Design review of the part built by this model. Coordinates are the model's own, in mm. Face numbers are marked on the shaded views. Give positions to 0.01 mm unless a question says otherwise; leave off trailing zeros. Order: outer loops, then holes, each group sorted by start corner. A loop starts at its lowest first (then second) coordinate and runs counter-clockwise, first axis right, second up. Notation, with made-up numbers: M 33.25,3 L 53.25,3 A8 ccw 53.25,10 Z; hole C 65.25,-2.75 d10. An arc over 180 degrees is marked long. Answer as a JSON object with one key per item and string values.
from build123d import *

# Parameters (mm, degrees)
SKETCH1_R           = 20
SKETCH1_R_2         = 1.5
SKETCH1_R_3         = 2
BOSS_EXTRUDE1_DEPTH = 7
SKETCH2_R           = 3.25
CUT_EXTRUDE1_DEPTH  = 1.5


with BuildPart() as part:
    # Sketch1 → Boss-Extrude1 (new body)
    with BuildSketch(Plane(origin=(0, 0, 0), x_dir=(1, 0, 0), z_dir=(0, 1, 0))):
        with Locations(Location((0, 0, 0), (0, 0, 270))):
            Circle(SKETCH1_R)
        with Locations(Location((0, 15.5, 0), (0, 0, 270))):
            Circle(SKETCH1_R_2, mode=Mode.SUBTRACT)
        with Locations(Location((15.5, 0, 0), (0, 0, 270))):
            Circle(SKETCH1_R_2, mode=Mode.SUBTRACT)
        with Locations(Location((0, -15.5, 0), (0, 0, 270))):
            Circle(SKETCH1_R_2, mode=Mode.SUBTRACT)
        with Locations(Location((-15.5, 0, 0), (0, 0, 270))):
            Circle(SKETCH1_R_2, mode=Mode.SUBTRACT)
        with Locations(Location((-4, 0, 0), (0, 0, 270))):
            Circle(SKETCH1_R_3, mode=Mode.SUBTRACT)
        with Locations(Location((4, 0, 0), (0, 0, 270))):
            Circle(SKETCH1_R_3, mode=Mode.SUBTRACT)
        with Locations(Location((0, 0, 0), (0, 0, 270))):
            Circle(SKETCH1_R_2, mode=Mode.SUBTRACT)
    extrude(amount=BOSS_EXTRUDE1_DEPTH)

    # Sketch2 → Cut-Extrude1 (cut)
    with BuildSketch(Plane(origin=(0, 7, 0), x_dir=(1, 0, 0), z_dir=(0, 1, 0))):
        with Locations(Location((0, 15.5, 0), (0, 0, 270))):
            Circle(SKETCH2_R)
        with Locations(Location((15.5, 0, 0), (0, 0, 270))):
            Circle(SKETCH2_R)
        with Locations(Location((0, -15.5, 0), (0, 0, 270))):
            Circle(SKETCH2_R)
        with Locations(Location((-15.5, 0, 0), (0, 0, 270))):
            Circle(SKETCH2_R)
    extrude(amount=-CUT_EXTRUDE1_DEPTH, mode=Mode.SUBTRACT)


solid = part.part
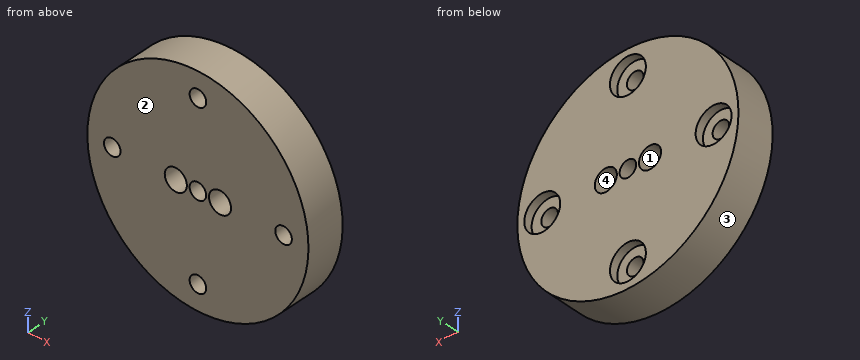
(1) To check wall thickness, follow L1, parallel to X at y = 2, z = 0; L2, parallel to Z at x = 2.5, y = 6.5; L3, parallel to X at y = 2.65, z = -15.5. State the ranges of each line that lie inside material, in increasing order. Write a range as from..to.
Checked values:
{"L1": "x = -20..-17, -14..-6, -2..-1.5, 1.5..2, 6..14, 17..20", "L2": "z = -19.84..-17.58, -13.42..-1.32, 1.32..13.42, 17.58..19.84", "L3": "x = -12.64..-1.5, 1.5..12.64"}
(2) We need section C-C (x = 0). Write out the cut boundary in (y, z).
Checked values:
{"outline": "M 0,-20 L 7,-20 L 7,-18.75 L 5.5,-18.75 L 5.5,-17 L 0,-17 Z; M 0,-14 L 5.5,-14 L 5.5,-12.25 L 7,-12.25 L 7,-1.5 L 0,-1.5 Z; M 0,1.5 L 7,1.5 L 7,12.25 L 5.5,12.25 L 5.5,14 L 0,14 Z; M 0,17 L 5.5,17 L 5.5,18.75 L 7,18.75 L 7,20 L 0,20 Z"}
(3) We need section B-B (z = 0). Count the separate pieces of the cut face and the enclosed holes in it, plus the area to 4 significant figures.
Checked values:
{"separate pieces": "6", "enclosed holes": "0", "area": "150.5 mm^2"}
(4) We need section A-A (y = 3.5). Write out the cut boundary in (x, z).
Checked values:
{"outline": "C 0,0 d40; hole C -15.5,0 d3; hole C -4,0 d4; hole C 0,-15.5 d3; hole C 0,0 d3; hole C 0,15.5 d3; hole C 4,0 d4; hole C 15.5,0 d3"}
(5) Draft analysis for pull direction Z (two halves, no side actions). For the marked faces 1, 2, 3 and 4, state which applies: +Z half, -Z half, draft (parallel to the pull), parting line (faces both ways), or undercut.
Checked values:
{"face 1": "undercut", "face 2": "draft", "face 3": "parting line", "face 4": "undercut"}
(6) We need section D-D (x = -5). Write out the cut boundary in (y, z), plus the area to 3 significant figures.
Checked values:
{"outline": "M 0,-19.36 L 7,-19.36 L 7,-1.73 L 0,-1.73 Z; M 0,1.73 L 7,1.73 L 7,19.36 L 0,19.36 Z", "area": "247 mm^2"}
(7) Insertion check: pin 1 (5 mm diameter, centred on x = -4, z = 0, fed in from +Y); pin 2 (2 mm diameter, centred on x = 14.5, z = 1, fed in from +Y); pin 3 (3 mm diameter, centred on y = 1, z = -6.5, fed in from +X); pin 4 (1 mm diameter, centred on x = -7, y = 3, fed in from -Z). Each pin has a flat end and moves straight along its axis. Give the tip position at first contact, or say it passes through.
Checked values:
{"pin 1": "stops at y = 7", "pin 2": "stops at y = 5.5", "pin 3": "stops at x = 19.36", "pin 4": "stops at z = -18.91"}
